Can you work these out from the model? Positions are in its coordinate system, mm. A direction names the side the tool comes from. Round coordinates to 2 decimals unless told otherwise and drop trailing zeros. Order: outer loops, then holes, each group sorted by start corner. A loop starts at its lowest first (then second) coordinate and runs counter-clockwise, first axis right, second up. Notation, with made-up numbers: (63, 72) -> (104, 72) arc R11 cw to (104, 83) -> close; hole circle Ø5 at (29, -12). An arc over 180 degrees is marked (long way). One line per item, written item: value.
```python
from build123d import *

# Parameters (mm, degrees)
F0_R     = 22.352
F1_DEPTH = 2.413
F3_R     = 18.0284006892
F4_DEPTH = 16.764
F5_R     = 1.27


# Not quite as in the source:
# - a fillet or chamfer that OpenCascade refuses, or shapes differently, is made with other operations: its cross-section is extruded or revolved along the edge and cut away or added


with BuildPart() as f1:
    # F0 (on Top) → F1 (new body)
    with BuildSketch(Plane.XY):
        Circle(F0_R)
    extrude(amount=F1_DEPTH)

    # F2: fillet of radius 5.08 on 1 edges, made by hand

    # F2_s1 → F2_t2 (revolve, cut)
    with BuildSketch(Plane.XZ):
        with BuildLine():
            ThreePointArc((22.352, 0), (20.5040864528, 1.7689192959), (18.0284006892, 2.413))
            Line((18.0284006892, 2.413), (22.352, 2.413))
            Line((22.352, 2.413), (22.352, 0))
        make_face()
    revolve(axis=Axis((0, 0, 2.413), (0, 0, 1)), mode=Mode.SUBTRACT)

    # F3 (on face) → F4 (join)
    with BuildSketch(Plane.XY.offset(2.413)):
        Circle(F3_R)
    extrude(amount=F4_DEPTH)

    # F5
    f5_edges = [f1.edges().sort_by_distance(p)[0] for p in [
        (-18.028401, 0, 19.177),
    ]]
    fillet(f5_edges, radius=F5_R)


solid = f1.part
```
Q1. Please list where these lines run through material, in increasing order: line 1 along Z through (x, y) = (6.5, -17); line 2 along Y through (x, z) = (-14.5, 10.5); line 3 along X through (y, z) = (10, 3.5).
Answers below:
line 1: 0 to 2.41
line 2: -10.71 to 10.71
line 3: -15 to 15
Q2. I want a section at C-C on z = 14. List the corners of the cut face in (x, y) for me, plus the area to 3 significant figures.
Answers below:
outline: circle Ø36.06 at (0, 0)
area: 1,020 mm^2
Q3. On a 3-axis mill with a long thin cutter (end or side, diameter ignored), from which of +Z, -Z, +X, -X, +Y, -Y can I reach the whole of each face in a straight line? I mean faces 1 (the face through (0, 0, 0)), 2 (the face through (-3.9, -17.6, 10.1)). Say none if no direction works.
Answers below:
face 1: -Z, +X, -X, +Y, -Y
face 2: +Z
Q4. Will these pins go through, and if not, where does the flat tip stop? pin 1 Ø1 at (x, z) = (7, 5.5) entering from -Y; pin 2 Ø5 at (x, z) = (6, 4) entering from +Y; pin 3 Ø1 at (y, z) = (1, 3.5) entering from +X; pin 4 Ø12 at (x, y) = (-17, -4) entering from -Z.
Answers below:
pin 1: y = -16.82
pin 2: y = 20.12
pin 3: x = 18.02
pin 4: z = 0
Q5. I want a section at A-A on x = 0. List the corners of the cut face in (y, z) for me, plus the area to 3 significant figures.
Answers below:
outline: (-22.35, 0) -> (22.35, 0) arc R5.08 ccw to (18.03, 2.41) -> (18.03, 17.91) arc R1.27 ccw to (16.76, 19.18) -> (-16.76, 19.18) arc R1.27 ccw to (-18.03, 17.91) -> (-18.03, 2.41) arc R5.08 ccw to start
area: 706 mm^2
